Source: CAD feature listing. Evaluate the final solid. Frame: model axes, mm. A direction names the side the tool comes from. Give positions to 0.01 mm unless a question says otherwise; leave off trailing zeros. Order: outer loops, then holes, each group sorted by start corner. A loop starts at its lowest first (then second) coordinate and runs counter-clockwise, first axis right, second up. Notation, with made-up numbers: M 36.5,72 L 93.5,72 A23 ccw 93.5,95 Z; hole C 71,61 d10. An arc over 180 degrees is marked long. Return JSON: item names as keys, results as strings.
from build123d import *

# Parameters (mm, degrees)
SKETCH3_R           = 5
BOSS_EXTRUDE1_DEPTH = 46
CUT_EXTRUDE1_DEPTH  = 300
CUT_EXTRUDE2_DEPTH  = 300
FILLET1_R           = 2


with BuildPart() as part:
    # Sketch3 → Boss-Extrude1 (new body)
    with BuildSketch(Plane.XY):
        with BuildLine():
            Line((40.883413809, 0), (3, 0))
            ThreePointArc((3, 0), (2.797908937, -1.891823319), (2.668267594, -3.789988061))
            ThreePointArc((2.668267594, -3.789988061), (6.682027739, -25.953006917), (20.054026368, -44.077557338))
            Line((20.054026368, -44.077557338), (64.595472348, -82.12438231))
            ThreePointArc((64.595472348, -82.12438231), (78.521745085, -83.314776326), (84.128579654, -70.511592488))
            Line((84.128579654, -70.511592488), (76.728855671, -56.958627104))
            Line((76.728855671, -56.958627104), (74.095757005, -58.396261068))
            Line((74.095757005, -58.396261068), (73.137334363, -56.640861957))
            Line((73.137334363, -56.640861957), (75.770433029, -55.203227993))
            Line((75.770433029, -55.203227993), (47.905010252, -4.166309429))
            ThreePointArc((47.905010252, -4.166309429), (44.9657217, -1.119973671), (40.883413809, 0))
        make_face()
        with Locations((72.389421761, -73)):
            Circle(SKETCH3_R, mode=Mode.SUBTRACT)
        with BuildLine():
            ThreePointArc((45.883413809, -8), (40.609242405, -12.992477345), (35.913481792, -7.452482191))
            ThreePointArc((35.913481792, -7.452482191), (41.157585213, -3.007522655), (45.883413809, -8))
        make_face(mode=Mode.SUBTRACT)
    extrude(amount=BOSS_EXTRUDE1_DEPTH)

    # Sketch4 → Cut-Extrude1 (cut)
    with BuildSketch(Plane(origin=(35.151571892, 19.192252189, 0), x_dir=(0, 0, -1), z_dir=(0.877699555, 0.479211321, 0))):
        Polygon((-40, -114.23699177), (-40, -70.47572427), (-33, -70.47572427), (-33, -18.71699177), (-13, -18.71699177), (-13, -70.47572427), (-6, -70.47572427), (-6, -114.23699177), align=None)
    extrude(amount=-CUT_EXTRUDE1_DEPTH, mode=Mode.SUBTRACT)

    # Sketch5 → Cut-Extrude2 (cut)
    with BuildSketch(Plane(origin=(0, 0, 0), x_dir=(1, 0, 0), z_dir=(0, 1, 0))):
        Polygon((39.057908144, -13), (27.904150662, -13), (27.904150662, -18), (20.883413809, -18), (20.883413809, -28), (26.883413809, -28), (26.883413809, -32.893409872), (39.057908144, -33), align=None)
    extrude(amount=-CUT_EXTRUDE2_DEPTH, mode=Mode.SUBTRACT)

    # Fillet1
    fillet1_edges = [part.edges().sort_by_distance(p)[0] for p in [
        (3, 0, 23),
    ]]
    fillet(fillet1_edges, radius=FILLET1_R)


solid = part.part
1. Draft query along Y for faces 5 (the face through (24, -4, 18)), 6 (the face through (14.178, -13.584, 23.14)), 7 (the face through (75.43, -57.67, 2.96)). Return one class per face: pulls with the +Y half, pulls with the -Y half, needs draft (parallel to the pull), parting line crosses it, or undercut.
Evaluation:
{"face 5": "needs draft", "face 6": "pulls with the -Y half", "face 7": "undercut"}
2. Ray query, probe 1 along Z at (x, y) = (60, -31); probe 2 along X at (y, z) = (-73, 2.8); probe 3 along X at (y, z) = (-11, 7). Return the intervals inside material, ascending.
Evaluation:
{"probe 1": "z = 0 to 13, 33 to 46", "probe 2": "x = 53.91 to 67.39, 77.39 to 84.39", "probe 3": "x = 2.84 to 36.88, 44.88 to 51.64"}
3. Set-up query: faces 1 (the face through (45.017, -1.151, 6.409)), 2 (the face through (53.73, -50.96, 36.55)), 3 (the face through (26.883, -3, 30)), 4 (the face through (74.44, -55.93, 42.96)). Return all of +Z, -Z, +X, -X, +Y, -Y with unobstructed straight access to the full face (end or side cutting, diameter ignored); none if empty.
Evaluation:
{"face 1": "+Z, -Z, +X, +Y", "face 2": "+X, -Y", "face 3": "+X, +Y, -Y", "face 4": "+Z, -Z, +X"}
4. Section query B-B (z = 36.5). Return loops of the section in (x, y), then the cut area to 3 significant figures.
Evaluation:
{"outline": "M 2.8,-1.82 A49.77 ccw 20.05,-44.08 L 38.1,-59.49 L 68.92,-42.66 L 47.91,-4.17 A8 ccw 40.88,0 L 4.8,0 A2 ccw Z; hole C 40.88,-8 d10", "area": "2,500 mm^2"}
5. First-contact query: pin 1 (11 mm diameter, centred on y = -3.5, z = 25, fed in from +X); pin 2 (12 mm diameter, centred on x = 49, z = 33.5, fed in from +Y); pin 3 (6 mm diameter, centred on y = -11, z = 36.5, fed in from -X); pin 4 (8 mm diameter, centred on x = 72.39, y = -73, fed in from -Z). Flat tips, straight axial feed; report the tip coordinate or a pass-through.
Evaluation:
{"pin 1": "stops at x = 26.88", "pin 2": "stops at y = -0.29", "pin 3": "stops at x = 2.64", "pin 4": "passes through"}
6. Section query A-A (y = -11). Return loops of the section in (x, z).
Evaluation:
{"outline": "M 2.84,0 L 36.88,0 L 36.88,13 L 18.91,13 L 18.91,33 L 36.88,33 L 36.88,46 L 2.84,46 Z; M 44.88,0 L 51.64,0 L 51.64,13 L 44.88,13 Z; M 44.88,33 L 51.64,33 L 51.64,46 L 44.88,46 Z"}
7. Section query D-D (y = -73). Return loops of the section in (x, z).
Evaluation:
{"outline": "M 53.91,0 L 67.39,0 L 67.39,6 L 53.91,6 Z; M 53.91,40 L 67.39,40 L 67.39,46 L 53.91,46 Z; M 77.39,0 L 84.39,0 L 84.39,6 L 77.39,6 Z; M 77.39,40 L 84.39,40 L 84.39,46 L 77.39,46 Z"}
8. Section query C-C (x = 29). Return loops of the section in (y, z).
Evaluation:
{"outline": "M -51.72,0 L 0,0 L 0,13 L -51.72,13 Z; M -51.72,33 L -5.49,33 L -5.49,32.91 L 0,32.91 L 0,46 L -51.72,46 Z"}
